CAD build for the part. Positions are in the model's coordinates, mm. Face numbers are marked on the shaded views. A direction names the side the tool comes from. Round coordinates to 2 decimals unless told otherwise and drop trailing zeros. Write each loop counter-clockwise with the first axis right and the second up, starting at its lowest first coordinate (ties: lowest second). Pieces come first, ordered by that corner, then holes. Notation, with made-up numbers: (-5.5, -17) - (8.5, -17) arc R20 cw to (8.5, 10) - close; hole circle Ø1 at (29, 11.5). An arc over 180 degrees is marked (long way). Use one line per item in the form item = value. Start each with the question number.
Item 1: Drill centre lines: L1, parallel to Y at x = 41, z = 2.75; L2, parallel to X at y = 15.5, z = 5.75; L3, parallel to X at y = -1, z = 6.5. Where is each one in solid material? Low to high.
Item 2: Tool access for the marked faces 1, 2 and 3: list every direction of +Z, -Z, +X, -X, +Y, -Y with a clear straight run to the whole face (end or side of a thin tool).
Item 3: Band-saw the part on C-C, the plane y = -14. List the corners of the cut face in (x, z).
Item 4: Band-saw the part on A-A, the plane z = 6.5. List the corners of the cut face in (x, y), and give its area (3 significant figures).
Item 5: Pin check, flat tips, straight feed: pin 1 (3 mm diameter, centred on x = 68, z = 6.5, fed in from -Y); pin 2 (5 mm diameter, centred on x = 54.5, z = 4.5, fed in from +Y); pin 3 (5 mm diameter, centred on y = -16, z = 4.5, fed in from +X). Stop position of each tip, or through.
Item 6: Band-saw the part on B-B, the plane x = 45. List the corners of the cut face in (y, z).
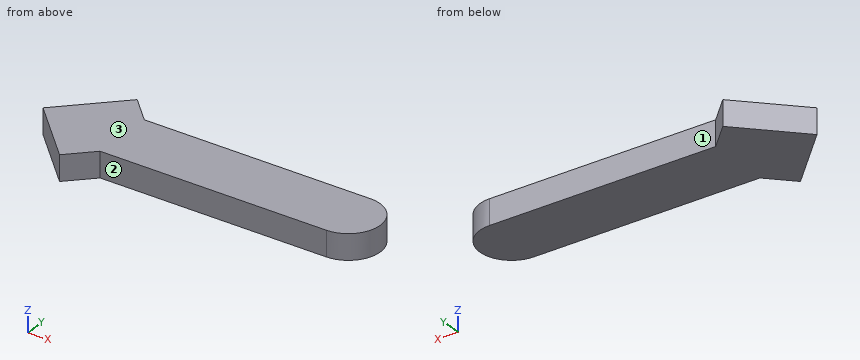
Autodesk Inventor part; units mm, degrees
ref_plane "YZ Plane" through (0, 0, 0) normal (1, 0, 0) x (0, 1, 0)
ref_plane "XZ Plane" through (0, 0, 0) normal (0, 1, 0) x (-1, 0, 0)
ref_plane "XY Plane" through (0, 0, 0) normal (0, 0, 1) x (1, 0, 0)
sketch "Sketch1" plane through (0, 0, 0) normal (0, 0, 1) x (1, 0, 0)
  line L0 (0, 21.9203) -> (21.9203, 0)
  line L1 (21.9203, 0) -> (0, -21.9203)
  line L2 (0, -21.9203) -> (-21.9203, 0)
  line L3 (-21.9203, 0) -> (0, 21.9203)
  line L4 (0, 12.5) -> (99, 12.5)
  arc A0 (99, -12.5) -> (99, 12.5) centre (99, 0) ccw
  line L5 (99, -12.5) -> (0, -12.5)
  line L6 (0, -12.5) -> (0, 12.5)
  point P0 (0, 0)
  point P1 (0, 0)
  point P2 (0, 0)
  dimension "d0" = 31
  dimension "d1" = 99
  dimension "d2" = 25
extrude "Extrusion1" add sketch "Sketch1" along normal blind 10
properties part number "layout aide"
Determined:
q1.L1 = -12.5 to 12.5
q1.L2 = -6.42 to 6.42
q1.L3 = -20.92 to 111.46
q2.face_1 = +Z, -Z, +X, +Y
q2.face_2 = +Z, -Z, +X, -Y
q2.face_3 = +Z, +X, -X, +Y, -Y
q3.outline = (-7.92, 0) - (7.92, 0) - (7.92, 10) - (-7.92, 10) - close
q4.outline = (-21.92, 0) - (0, -21.92) - (9.42, -12.5) - (99, -12.5) arc R12.5 ccw to (99, 12.5) - (9.42, 12.5) - (0, 21.92) - close
q4.area = 3,290 mm²
q5.pin_1 = -12.5
q5.pin_2 = 12.5
q5.pin_3 = 8.42
q6.outline = (-12.5, 0) - (12.5, 0) - (12.5, 10) - (-12.5, 10) - close
